The listing builds one solid part. Answer for the finished solid, in the listing's coordinates (mm). A direction names the side the tool comes from. Coordinates: 2 decimals unless noted, no trailing zeros. Loops run counter-clockwise (first coordinate to the right, second up) from the corner with the lowest first, then second, coordinate; pieces in that order, holes last. Notation, with made-up numbers: (16.25, 61.5) - (74.25, 61.5) arc R19 cw to (74.25, 93.5) - close; hole circle Ø4 at (3, -5.75). An arc over 180 degrees is marked (long way). Put each result on its own line as item: value.
```python
from build123d import *

# Parameters (mm, degrees)
SKETCH1_R           = 28.575
BOSS_EXTRUDE1_DEPTH = 10
SKETCH2_R           = 19.05
CUT_EXTRUDE1_DEPTH  = 11
SKETCH5_R           = 2.25
CUT_EXTRUDE2_DEPTH  = 58.15
SKETCH6_R           = 2.25
CUT_EXTRUDE3_DEPTH  = 11.0000001
CUT_EXTRUDE5_START  = -10
SKETCH7_R           = 4
SKETCH7_R_2         = 2.25
CUT_EXTRUDE5_DEPTH  = 4
CUT_EXTRUDE6_START  = -47.15
SKETCH7_4_R         = 4
SKETCH7_4_R_2       = 2.25
CUT_EXTRUDE6_DEPTH  = 4
CIRPATTERN6_COUNT   = 2
CIRPATTERN6_ANGLE   = 90


with BuildPart() as part:
    # Sketch1 → Boss-Extrude1 (new body)
    with BuildSketch(Plane.XY):
        Circle(SKETCH1_R)
    extrude(amount=BOSS_EXTRUDE1_DEPTH)

    # Sketch2 → Cut-Extrude1 (cut, through all)
    with BuildSketch(Plane.XY.offset(10)):
        Circle(SKETCH2_R)
    extrude(amount=-CUT_EXTRUDE1_DEPTH, mode=Mode.SUBTRACT)

    # Sketch5 → Cut-Extrude2 (cut, through all)
    with BuildSketch(Plane(origin=(0, 28.575, 0), x_dir=(1, 0, 0), z_dir=(0, 1, 0))):
        with Locations((0, -5)):
            Circle(SKETCH5_R)
    cut_extrude2 = extrude(amount=-CUT_EXTRUDE2_DEPTH, mode=Mode.SUBTRACT)

    # Sketch6 → Cut-Extrude3 (cut, through all)
    with BuildSketch(Plane.XY.offset(10)):
        with Locations((-16.970562748, 16.970562748)):
            Circle(SKETCH6_R)
        with Locations((16.970562748, 16.970562748)):
            Circle(SKETCH6_R)
        with Locations((16.970562748, -16.970562748)):
            Circle(SKETCH6_R)
        with Locations((-16.970562748, -16.970562748)):
            Circle(SKETCH6_R)
    extrude(amount=-CUT_EXTRUDE3_DEPTH, mode=Mode.SUBTRACT)

    # Sketch7 → Cut-Extrude5 (cut)
    with BuildSketch(Plane(origin=(0, 28.575, 0), x_dir=(1, 0, 0), z_dir=(0, 1, 0)).offset(CUT_EXTRUDE5_START)):
        with Locations((0, -5)):
            Circle(SKETCH7_R)
        with Locations((0, -5)):
            Circle(SKETCH7_R_2, mode=Mode.SUBTRACT)
    cut_extrude5 = extrude(amount=CUT_EXTRUDE5_DEPTH, mode=Mode.SUBTRACT)

    # Sketch7<4> → Cut-Extrude6 (cut)
    with BuildSketch(Plane(origin=(0, 28.575, 0), x_dir=(1, 0, 0), z_dir=(0, 1, 0)).offset(CUT_EXTRUDE6_START)):
        with Locations((0, -5)):
            Circle(SKETCH7_4_R)
        with Locations((0, -5)):
            Circle(SKETCH7_4_R_2, mode=Mode.SUBTRACT)
    cut_extrude6 = extrude(amount=-CUT_EXTRUDE6_DEPTH, mode=Mode.SUBTRACT)

    # CirPattern6: Cut-Extrude2, Cut-Extrude5, Cut-Extrude6 ×2 about axis
    cirpattern6_axis = Axis((0, 0, 10), (0, 0, 1))
    for i in range(1, CIRPATTERN6_COUNT):
        add(cut_extrude2.rotate(cirpattern6_axis, i * CIRPATTERN6_ANGLE / (CIRPATTERN6_COUNT - 1)), mode=Mode.SUBTRACT)
        add(cut_extrude5.rotate(cirpattern6_axis, i * CIRPATTERN6_ANGLE / (CIRPATTERN6_COUNT - 1)), mode=Mode.SUBTRACT)
        add(cut_extrude6.rotate(cirpattern6_axis, i * CIRPATTERN6_ANGLE / (CIRPATTERN6_COUNT - 1)), mode=Mode.SUBTRACT)


solid = part.part
```
1) Each of these flat-tipped pins is pushed along its axis until it touches: pin 1 (2.5 mm diameter, centred on x = -16.97, y = -16.97, fed in from +Z); pin 2 (2 mm diameter, centred on x = 11, z = 1.5, fed in from +Y); pin 3 (3 mm diameter, centred on y = -6, z = 2, fed in from -X); pin 4 (3 mm diameter, centred on x = -23, z = 6, fed in from -Y). Where does it stop, or does it pass through?
Found:
pin 1: passes through
pin 2: stops at y = 26.77
pin 3: stops at x = -28.22
pin 4: stops at y = -18.82
2) For faces 1 (the face through (2, 22.575, 7)), 2 (the face through (-25.617, -0.488, 7.196)), determine the directions among +Z, -Z, +X, -X, +Y, -Y from which every point of the face is accessible in a straight line to the end or side of a thin tool.
Found:
face 1: none
face 2: +X, -X
3) For a pull along Z with two mould halves and no side action, classify faces 3 (the face through (6, -19, 10)), 4 (the face through (-20.573, -0.867, 8.905)), 5 (the face through (18.009, -18.967, 5.07)) as pulls with the +Z half, pulls with the -Z half, needs draft (parallel to the pull), parting line crosses it, or undercut.
Found:
face 3: pulls with the +Z half
face 4: undercut
face 5: needs draft
4) The part is cut by section A-A (x = 0). Give the vertices of the cut face in (y, z) (3 decimals).
Found:
outline: (-28.575, 0) - (-19.05, 0) - (-19.05, 1) - (-22.575, 1) - (-22.575, 2.75) - (-28.575, 2.75) - close; (-28.575, 7.25) - (-22.575, 7.25) - (-22.575, 9) - (-19.05, 9) - (-19.05, 10) - (-28.575, 10) - close; (19.05, 0) - (28.575, 0) - (28.575, 2.75) - (22.575, 2.75) - (22.575, 1) - (19.05, 1) - close; (19.05, 9) - (22.575, 9) - (22.575, 7.25) - (28.575, 7.25) - (28.575, 10) - (19.05, 10) - close
5) The part is cut by section C-C (y = -13). Give the vertices of the cut face in (x, z).
Found:
outline: (-25.45, 0) - (-13.92, 0) - (-13.92, 10) - (-25.45, 10) - close; (13.92, 0) - (25.45, 0) - (25.45, 10) - (13.92, 10) - close
6) Straight lines are drawn through the part: L1, parallel to X at y = 15.5, z = 9.75; L2, parallel to Z at x = 26, y = 0; L3, parallel to Z at x = 21.2, y = 0. For each, find the intervals that lie inside material, in ascending order. Write a range as [from, to].
Found:
L1: x = [-24.01, -18.67], [-15.27, -11.07], [11.07, 15.27], [18.67, 24.01]
L2: z = [0, 2.75], [7.25, 10]
L3: z = [0, 1], [9, 10]
7) The part is cut by section D-D (x = -11.5). Give the vertices of the cut face in (y, z), and give its area (3 significant figures).
Found:
outline: (-26.16, 0) - (-15.19, 0) - (-15.19, 10) - (-26.16, 10) - close; (15.19, 0) - (26.16, 0) - (26.16, 10) - (15.19, 10) - close
area: 219 mm^2
